For this review, take the finished solid that the model builds, in its own axes (mm). A direction names the side the tool comes from. Give positions to 0.01 mm unless a question says otherwise; leave off trailing zeros. Loops run counter-clockwise (first coordinate to the right, second up) from the corner with the lowest first, then second, coordinate; pieces in that order, holes last. Notation, with made-up numbers: (25, 22.5) - (79, 22.5) arc R19 cw to (79, 31.5) - close; hole circle Ø3 at (-10, -35). An arc over 180 degrees is marked (long way). Answer as CSV lines item,"result".
from build123d import *

# Parameters (mm, degrees)
SKETCH4_W               = 296
SKETCH4_H               = 10.8
CUT_EXTRUDE1_DEPTH      = 11.8
CUT_EXTRUDE1_DEPTH_BACK = 11.8
SKETCH2_R               = 3.97
EXTRUDE2_DEPTH          = 30.6
SKETCH3_R               = 3.97
EXTRUDE3_DEPTH          = 30.6


with BuildPart() as part:
    # Sketch4 → Revolve1 (revolve)
    with BuildSketch(Plane.XY):
        with Locations((0, 5.4)):
            Rectangle(SKETCH4_W, SKETCH4_H)
    revolve(axis=Axis((-180.472392976, 0, 0), (1, 0, 0)))

    # Sketch5 → Cut-Extrude1 (cut, two sides)
    with BuildSketch(Plane(origin=(0, 0, 0), x_dir=(1, 0, 0), z_dir=(0, 1, 0))) as cut_extrude1_sk:
        Polygon((-172.80595371, 7.9), (-135, 7.9), (-126.264796731, 16.635203269), (-172.80595371, 16.635203269), align=None)
        Polygon((-172.80595371, -7.9), (-135, -7.9), (-126.264796731, -16.635203269), (-172.80595371, -16.635203269), align=None)
        Polygon((135, -7.9), (126.264796731, -16.635203269), (172.80595371, -16.635203269), (172.80595371, -7.9), align=None)
        Polygon((135, 7.9), (126.264796731, 16.635203269), (172.80595371, 16.635203269), (172.80595371, 7.9), align=None)
    extrude(amount=CUT_EXTRUDE1_DEPTH, mode=Mode.SUBTRACT)
    extrude(cut_extrude1_sk.sketch, amount=-CUT_EXTRUDE1_DEPTH_BACK, mode=Mode.SUBTRACT)

    # Sketch2 → Extrude2 (cut)
    with BuildSketch(Plane(origin=(-148, 0, 0), x_dir=(0, 0, -1), z_dir=(1, 0, 0))):
        Circle(SKETCH2_R)
    extrude(amount=EXTRUDE2_DEPTH, mode=Mode.SUBTRACT)

    # Sketch3 → Extrude3 (cut)
    with BuildSketch(Plane.ZY.offset(-148)):
        Circle(SKETCH3_R)
    extrude(amount=EXTRUDE3_DEPTH, mode=Mode.SUBTRACT)


solid = part.part
1) Wall thickness on line 1 (Y direction, x = -130.5, z = 0); line 2 (Y direction, x = 98.5, z = 1); line 3 (Z direction, x = -30.5, y = -0.25): over which ranges is each line inside the solid? List them lowest first. Write a range as from..to.
From the geometry:
line 1,"y = -10.8..-3.97, 3.97..10.8"
line 2,"y = -10.75..10.75"
line 3,"z = -10.8..10.8"
2) Consider section B-B on z = 0. Write out the cut boundary in (x, y), and give its area (3 significant figures).
From the geometry:
outline,"(-148, -10.8) - (148, -10.8) - (148, -3.97) - (117.4, -3.97) - (117.4, 3.97) - (148, 3.97) - (148, 10.8) - (-148, 10.8) - (-148, 3.97) - (-117.4, 3.97) - (-117.4, -3.97) - (-148, -3.97) - close"
area,"5,910 mm^2"
3) Draft analysis for pull direction Y (two halves, no side actions). For faces 6 (the flat face through (-142, 0, 7.9)), 7 (the cylindrical face through (2.072, -1.406, 10.708)), 8 (the cylindrical face through (-132.914, 1.192, -3.787)), state which applies: pulls with the +Y half, pulls with the -Y half, needs draft (parallel to the pull), parting line crosses it, or undercut.
From the geometry:
face 6,"needs draft"
face 7,"parting line crosses it"
face 8,"undercut"
4) Consider section C-C on x = 36.5. Write out the cut boundary in (y, z).
From the geometry:
outline,"circle Ø21.6 at (0, 0)"
5) Machinability: for faces 1 (the flat face through (142, 0, 7.9)), 2 (the cylindrical face through (132.914, 1.192, 3.787)), 3 (the flat face through (142, 0, -7.9)), 4 (the flat face through (-117.4, 0, 0)), 5 (the flat face through (-142, 0, -7.9)), which of the approach directions +Z, -Z, +X, -X, +Y, -Y give a long, thin tool a straight path to every point of the face, cutting with its end or side? Answer none if there is none.
From the geometry:
face 1,"+Z, +X, +Y, -Y"
face 2,"+X"
face 3,"-Z, +X, +Y, -Y"
face 4,"-X"
face 5,"-Z, -X, +Y, -Y"
6) Insertion check: P1, Ø6.5, axis at x = -139.5, y = 1.5, coming from the -Z side; P2, Ø4, axis at x = 33, y = -5, coming from the +Z side; P3, Ø1, axis at x = 39, z = 3.5, coming from the +Y side. Each pin has a flat end and moves straight along its axis. Give the tip position at first contact, or say it passes through.
From the geometry:
P1,"stops at z = -7.9"
P2,"stops at z = 10.37"
P3,"stops at y = 10.37"
7) Consider section A-A on y = 0. Write out the cut boundary in (x, z).
From the geometry:
outline,"(-148, -7.9) - (-135, -7.9) - (-132.1, -10.8) - (132.1, -10.8) - (135, -7.9) - (148, -7.9) - (148, -3.97) - (117.4, -3.97) - (117.4, 3.97) - (148, 3.97) - (148, 7.9) - (135, 7.9) - (132.1, 10.8) - (-132.1, 10.8) - (-135, 7.9) - (-148, 7.9) - (-148, 3.97) - (-117.4, 3.97) - (-117.4, -3.97) - (-148, -3.97) - close"
